Drawing for the job (mm, zero at the part's lowest x, y, z). A direction names the side the tool comes from. Round coordinates to 2 decimals unless told otherwise and drop trailing zeros. Write each loop counter-clockwise with the first axis right and the second up, starting at its lowest first coordinate (ties: lowest second). Pieces come first, ordered by that corner, then holes.
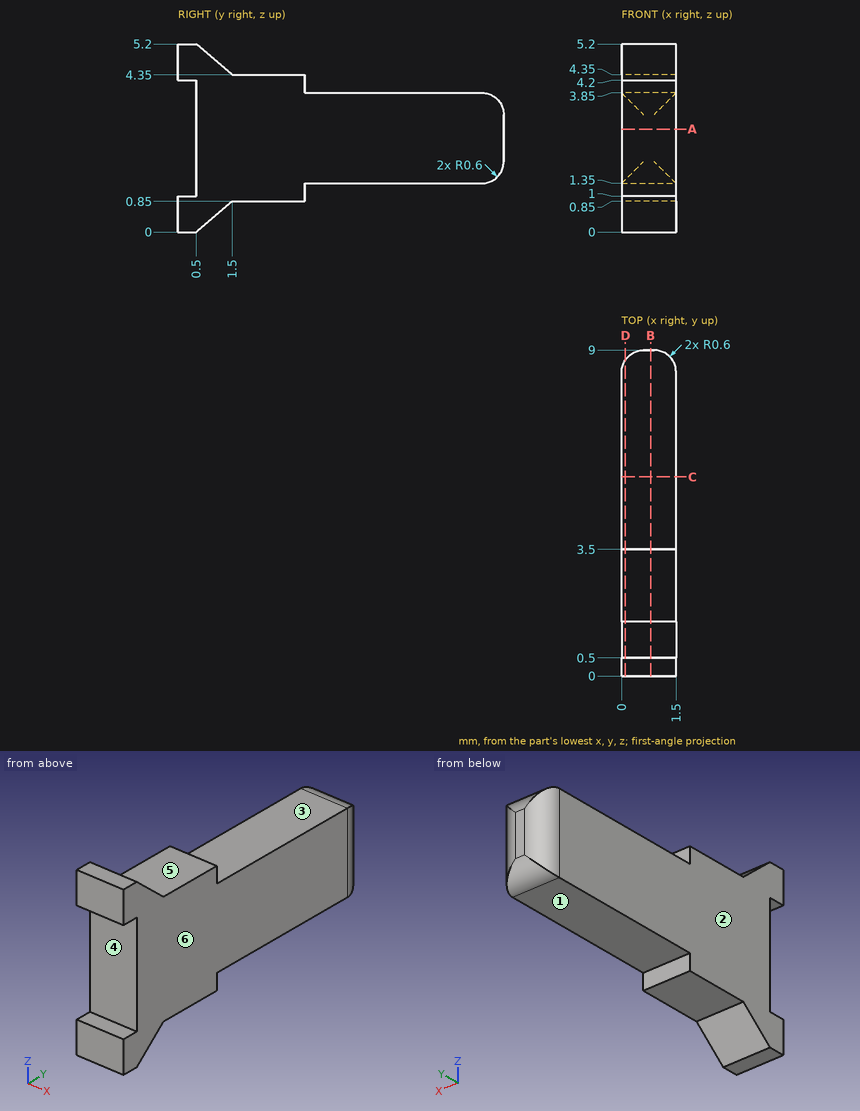
Q1. Tool access for the marked faces 1, 2 and 3: list every direction of +Z, -Z, +X, -X, +Y, -Y with a clear straight run to the whole face (end or side of a thin tool).
Q2. Wall check: line 1 (Z direction, x = 0.7, y = 6.25); line 2 (Z direction, x = 0.35, y = 2.5); line 3 (Y direction, x = 0.6, z = 2.1). Give the ranges that are in metal, low to high.
Q3. Saw through at C-C, the plane y = 5.5. Write the cut outline in (x, z).
Q4. Saw through at D-D, the plane x = 0.1. Write the cut outline in (y, z), and give its area (3 significant figures).
Q5. Saw through at B-B, the plane x = 0.8. Write the cut outline in (y, z).
Q6. Drop a flat-ended pin along its axis: P1, Ø0.8, axis at x = 1, y = 7, coming from the -Z side. Give the stop position or say it passes through.
Q7. Two-plate mould, pull along Z, no slides. Class the marked faces 4, 5 and 6: released by +Z, released by -Z, zero draft, split by the parting line, or undercut.
Q8. Saw through at A-A, the plane z = 2.85. Write the cut outline in (x, y).
Computed:
1. face 1: -Z, +X, -X, +Y
1. face 2: +Z, -Z, -X, +Y, -Y
1. face 3: +Z, +X, -X, +Y
2. line 1: z = 1.35 to 3.85
2. line 2: z = 0.85 to 4.35
2. line 3: y = 0.5 to 9
3. outline: (0, 1.35) - (1.5, 1.35) - (1.5, 3.85) - (0, 3.85) - close
4. outline: (0, 0) - (0.5, 0) - (1.5, 0.85) - (3.5, 0.85) - (3.5, 1.35) - (8.4, 1.35) arc R0.6 ccw to (8.73, 1.45) - (8.73, 3.75) arc R0.6 ccw to (8.4, 3.85) - (3.5, 3.85) - (3.5, 4.35) - (1.5, 4.35) - (0.5, 5.2) - (0, 5.2) - (0, 4.2) - (0.5, 4.2) - (0.5, 1) - (0, 1) - close
4. area: 25.4 mm2
5. outline: (0, 0) - (0.5, 0) - (1.5, 0.85) - (3.5, 0.85) - (3.5, 1.35) - (8.4, 1.35) arc R0.6 ccw to (9, 1.95) - (9, 3.25) arc R0.6 ccw to (8.4, 3.85) - (3.5, 3.85) - (3.5, 4.35) - (1.5, 4.35) - (0.5, 5.2) - (0, 5.2) - (0, 4.2) - (0.5, 4.2) - (0.5, 1) - (0, 1) - close
6. P1: stops at z = 1.35
7. face 4: undercut
7. face 5: released by +Z
7. face 6: zero draft
8. outline: (0, 0.5) - (1.5, 0.5) - (1.5, 8.4) arc R0.6 ccw to (0.9, 9) - (0.6, 9) arc R0.6 ccw to (0, 8.4) - close
